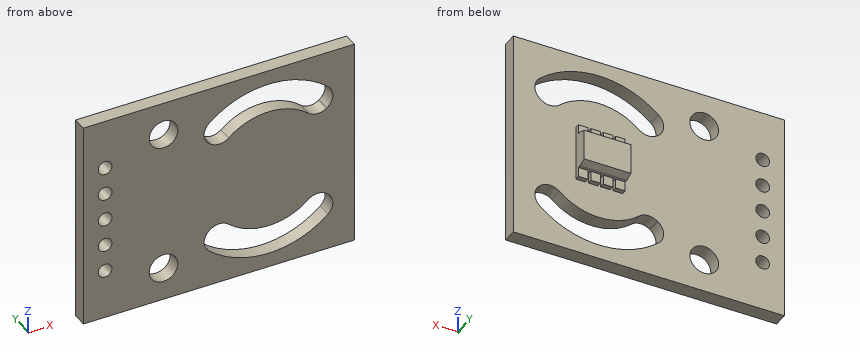
```python
from build123d import *

# Parameters (mm, degrees)
SKETCH1_W             = 28.4
SKETCH1_H             = 22
BOSS_EXTRUDE1_DEPTH   = 1.5
SKETCH2_R             = 1.5
SKETCH2_R_2           = 0.72
CUT_EXTRUDE1_DEPTH    = 2.5
FILLET1_R             = 1.5
SKETCH3_W             = 4.9
SKETCH3_H             = 3.8
BOSS_EXTRUDE2_DEPTH   = 1.6
CHAMFER1_SIZE         = 0.8
CHAMFER1_SIZE2        = 0.291176187
CHAMFER1_PART_2_SIZE  = 0.8
CHAMFER1_PART_2_SIZE2 = 0.291176187
SKETCH6_W             = 1
SKETCH6_H             = 1
BOSS_EXTRUDE3_DEPTH   = 0.5


with BuildPart() as part:
    # Sketch1 → Boss-Extrude1 (new body)
    with BuildSketch(Plane(origin=(0, 0, 0), x_dir=(1, 0, 0), z_dir=(0, 1, 0))):
        Rectangle(SKETCH1_W, SKETCH1_H)
    extrude(amount=BOSS_EXTRUDE1_DEPTH)

    # Sketch2 → Cut-Extrude1 (cut, through all)
    with BuildSketch(Plane(origin=(0, 1.5, 0), x_dir=(1, 0, 0), z_dir=(0, 1, 0))):
        with Locations(Location((-5.8, 7.5, 0), (0, 0, 270))):  # turned: the seam where the file's is
            Circle(SKETCH2_R)
        with Locations(Location((-5.8, -7.5, 0), (0, 0, 270))):  # turned: the seam where the file's is
            Circle(SKETCH2_R)
        with Locations(Location((-11.92285327, 5.76, 0), (0, 0, 270))):  # turned: the seam where the file's is
            Circle(SKETCH2_R_2)
        with Locations(Location((-11.92285327, 2.88, 0), (0, 0, 270))):  # turned: the seam where the file's is
            Circle(SKETCH2_R_2)
        with Locations(Location((-11.92285327, 0, 0), (0, 0, 270))):  # turned: the seam where the file's is
            Circle(SKETCH2_R_2)
        with Locations(Location((-11.92285327, -2.88, 0), (0, 0, 270))):  # turned: the seam where the file's is
            Circle(SKETCH2_R_2)
        with Locations(Location((-11.92285327, -5.76, 0), (0, 0, 270))):  # turned: the seam where the file's is
            Circle(SKETCH2_R_2)
        with BuildLine():
            Line((-2.3, 5.830951895), (0.2, 3.994996871))
            ThreePointArc((0.2, 3.994996871), (5.2, 6.4), (10.2, 3.994996871))
            Line((10.2, 3.994996871), (12.7, 5.830951895))
            ThreePointArc((12.7, 5.830951895), (5.2, 9.5), (-2.3, 5.830951895))
        make_face()
        with BuildLine():
            Line((10.2, -3.994996871), (12.7, -5.830951895))
            ThreePointArc((12.7, -5.830951895), (5.2, -9.5), (-2.3, -5.830951895))
            Line((-2.3, -5.830951895), (0.2, -3.994996871))
            ThreePointArc((0.2, -3.994996871), (5.2, -6.4), (10.2, -3.994996871))
        make_face()
    extrude(amount=-CUT_EXTRUDE1_DEPTH, mode=Mode.SUBTRACT)

    # Fillet1
    fillet1_edges = [part.edges().sort_by_distance(p)[0] for p in [
        (-2.3, 0.75, -5.830951895),
        (12.7, 0.75, -5.830951895),
        (10.2, 0.75, -3.994996871),
        (0.2, 0.75, -3.994996871),
        (0.2, 0.75, 3.994996871),
        (10.2, 0.75, 3.994996871),
        (12.7, 0.75, 5.830951895),
        (-2.3, 0.75, 5.830951895),
    ]]
    fillet(fillet1_edges, radius=FILLET1_R)

    # Sketch3 → Boss-Extrude2 (add)
    with BuildSketch(Plane(origin=(0, 1.5, 0), x_dir=(1, 0, 0), z_dir=(0, 1, 0))):
        with Locations((5.2, 0)):
            Rectangle(SKETCH3_W, SKETCH3_H)
    extrude(amount=BOSS_EXTRUDE2_DEPTH)

    # Chamfer1
    chamfer1_edges = [part.edges().sort_by_distance(p)[0] for p in [
        (5.2, 3.1, 1.9),
    ]]
    chamfer1_side = [part.faces().sort_by_distance(p)[0] for p in [
        (5.2, 2.3, 1.9),
    ]]
    chamfer(chamfer1_edges, length=CHAMFER1_SIZE, length2=CHAMFER1_SIZE2, reference=chamfer1_side[0])

    # Chamfer1 part 2
    chamfer1_part_2_edges = [part.edges().sort_by_distance(p)[0] for p in [
        (5.2, 3.1, -1.9),
    ]]
    chamfer1_part_2_side = [part.faces().sort_by_distance(p)[0] for p in [
        (5.2, 2.3, -1.9),
    ]]
    chamfer(chamfer1_part_2_edges, length=CHAMFER1_PART_2_SIZE, length2=CHAMFER1_PART_2_SIZE2, reference=chamfer1_part_2_side[0])

    # Sketch6 → Boss-Extrude3 (add)
    with BuildSketch(Plane(origin=(0, 1.5, 0), x_dir=(1, 0, 0), z_dir=(0, 1, 0))):
        with Locations((3.25, -2.4)):
            Rectangle(SKETCH6_W, SKETCH6_H)
        with Locations((3.25, 2.4)):
            Rectangle(SKETCH6_W, SKETCH6_H)
        with Locations((4.55, -2.4)):
            Rectangle(SKETCH6_W, SKETCH6_H)
        with Locations((4.55, 2.4)):
            Rectangle(SKETCH6_W, SKETCH6_H)
        with Locations((5.85, -2.4)):
            Rectangle(SKETCH6_W, SKETCH6_H)
        with Locations((5.85, 2.4)):
            Rectangle(SKETCH6_W, SKETCH6_H)
        with Locations((7.15, -2.4)):
            Rectangle(SKETCH6_W, SKETCH6_H)
        with Locations((7.15, 2.4)):
            Rectangle(SKETCH6_W, SKETCH6_H)
    extrude(amount=BOSS_EXTRUDE3_DEPTH)


solid = part.part
```
CAD build for the part. Positions are in the model's coordinates, mm. Give positions to 0.01 mm unless a question says otherwise; leave off trailing zeros. Write each loop counter-clockwise with the first axis right and the second up, starting at its lowest first coordinate (ties: lowest second). Pieces come first, ordered by that corner, then holes. Notation, with made-up numbers: M 70,-22 L 89,-22 A29 cw 89,14 Z; hole C -25.75,14.5 d7. An arc over 180 degrees is marked long. Return JSON: item names as keys, results as strings. Group by question number.
(1) Band-saw the part on D-D (x = -9). Give the cut face in (y, z).
(2) Band-saw the part on C-C (z = -7.5). Give the cut face in (x, y), and give its area (3 significant figures).
(3) Band-saw the part on B-B (x = -5.8). Give the cut face in (y, z).
(4) Drill centre lines: L1, parallel to X at y = 1.05, z = 0; L2, parallel to Z at x = -7, y = 0.45; L3, parallel to X at y = 1, z = 5.25. Where is each one in solid material? Low to high. Write a range as [from, to].
(5) Flat gauge pins, fed straight in: pin 1 Ø0.6 at (x, y) = (6, 2) entering from -Z; pin 2 Ø0.8 at (y, z) = (2, -1) entering from -X; pin 3 Ø1.9 at (x, z) = (-11.92, -5.76) entering from +Y; pin 4 Ø6 at (x, z) = (9, 2.5) entering from +Y. Where does each tip first touch, or does it go through?
(6) Band-saw the part on A-A (z = 0). Give the cut face in (x, y), and give its area (3 significant figures).
Entries:
{
 "1": {"outline": "M 0,-11 L 1.5,-11 L 1.5,11 L 0,11 Z"},
 "2": {"outline": "M -14.2,0 L -7.3,0 L -7.3,1.5 L -14.2,1.5 Z; M -4.3,0 L -0.63,0 L -0.63,1.5 L -4.3,1.5 Z; M 11.03,0 L 14.2,0 L 14.2,1.5 L 11.03,1.5 Z", "area": "20.6 mm^2"},
 "3": {"outline": "M 0,-11 L 1.5,-11 L 1.5,-9 L 0,-9 Z; M 0,-6 L 1.5,-6 L 1.5,6 L 0,6 Z; M 0,9 L 1.5,9 L 1.5,11 L 0,11 Z"},
 "4": {"L1": "x = [-14.2, -12.64], [-11.2, 14.2]", "L2": "z = [-11, -8.4], [-6.6, 6.6], [8.4, 11]", "L3": "x = [-14.2, -12.43], [-11.41, -1.32], [1.54, 8.86], [11.72, 14.2]"},
 "5": {"pin 1": "stops at z = -2.9", "pin 2": "stops at x = 2.75", "pin 3": "stops at y = 1.5", "pin 4": "stops at y = 3.1"},
 "6": {"outline": "M -14.2,0 L -12.64,0 L -12.64,1.5 L -14.2,1.5 Z; M -11.2,0 L 14.2,0 L 14.2,1.5 L 7.65,1.5 L 7.65,3.1 L 2.75,3.1 L 2.75,1.5 L -11.2,1.5 Z", "area": "48.3 mm^2"}
}
